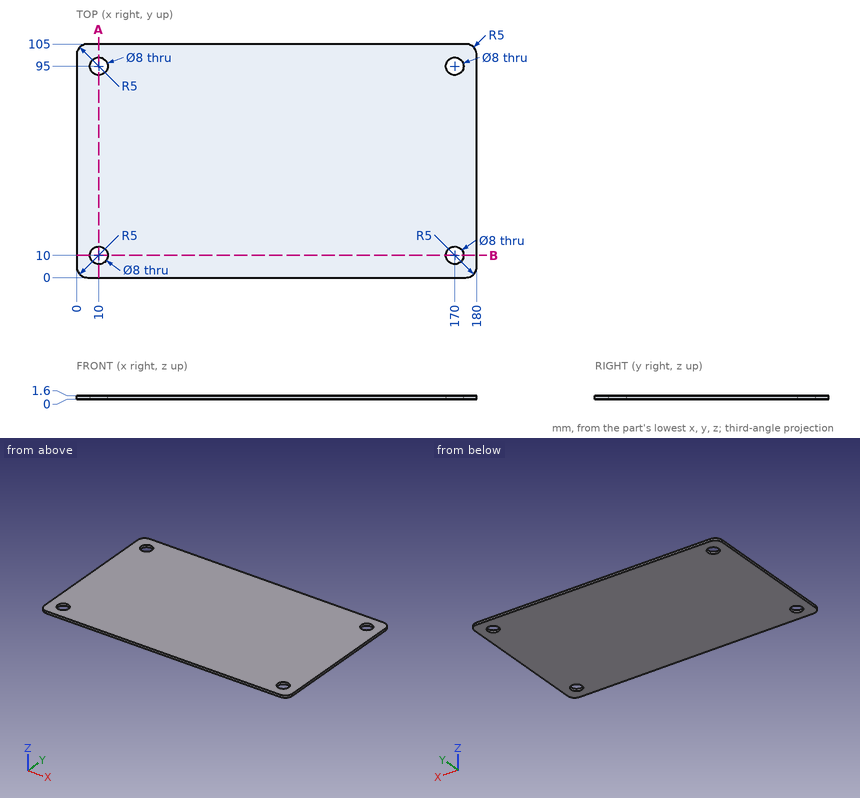
Part print with two shaded views. Sizes in mm from the minimum x, y, z corner. Coordinates: 2 decimals unless noted, no trailing zeros. Write each loop counter-clockwise with the first axis right and the second up, starting at its lowest first coordinate (ties: lowest second). Pieces come first, ordered by that corner, then holes.
(1) Pin check, flat tip, straight feed: pin 1 Ø5 at (x, y) = (10, 10) entering from -Z. Stop position of the tip, or through.
(2) Cut at A-A on x = 10. List the corners of the cut face in (y, z), and give its area (3 significant figures).
(3) Drill centre lines: line 1 (Y direction, x = 10, z = 0.7); line 2 (X direction, y = 95, z = 0.8); line 3 (Y direction, x = 11.5, z = 0.4). Where is each one in solid material? Low to high.
(4) Cut at B-B on y = 10. List the corners of the cut face in (x, z), and give its area (3 significant figures).
Working result:
1. pin 1: passes through
2. outline: (0, 0) - (6, 0) - (6, 1.6) - (0, 1.6) - close; (14, 0) - (91, 0) - (91, 1.6) - (14, 1.6) - close; (99, 0) - (105, 0) - (105, 1.6) - (99, 1.6) - close
2. area: 142 mm2
3. line 1: y = 0 to 6, 14 to 91, 99 to 105
3. line 2: x = 0 to 6, 14 to 166, 174 to 180
3. line 3: y = 0 to 6.29, 13.71 to 91.29, 98.71 to 105
4. outline: (0, 0) - (6, 0) - (6, 1.6) - (0, 1.6) - close; (14, 0) - (166, 0) - (166, 1.6) - (14, 1.6) - close; (174, 0) - (180, 0) - (180, 1.6) - (174, 1.6) - close
4. area: 262 mm2
